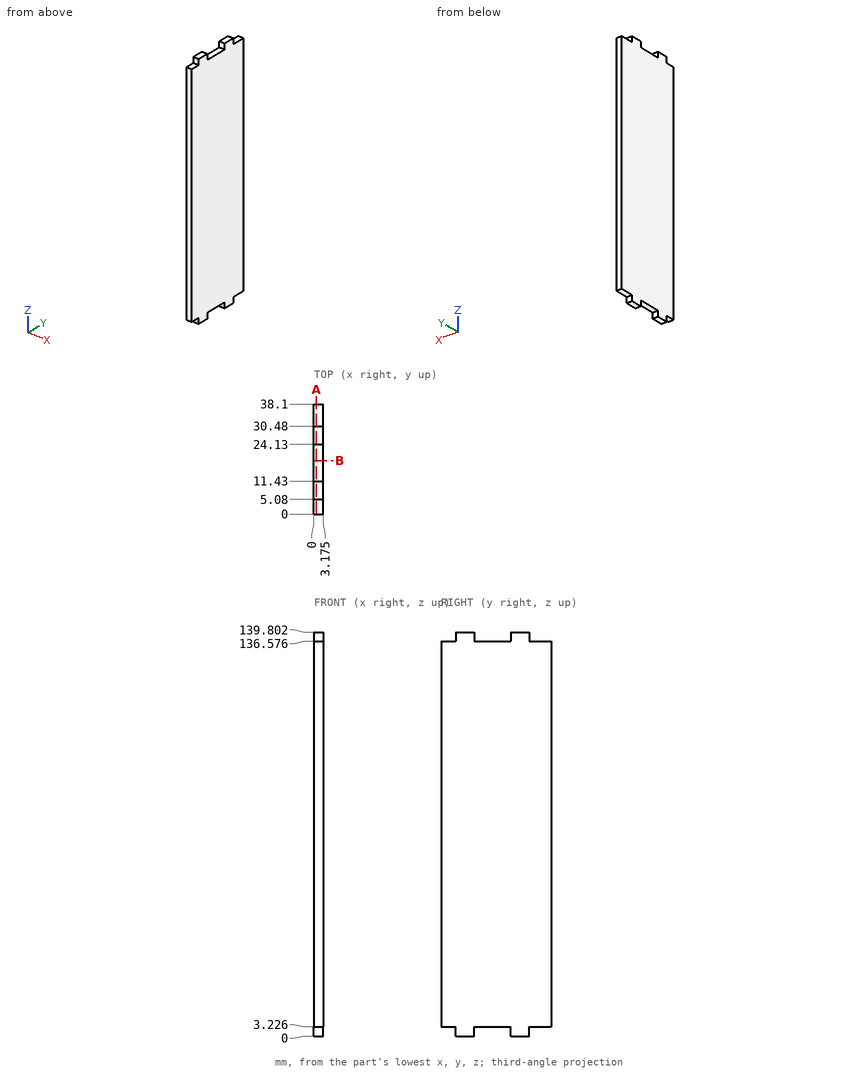
Geometry check sheet. Reference: drawing and pictorial views, mm from the part's lowest x, y, z. Give positions to 0.01 mm unless a question says otherwise; leave off trailing zeros. Loops run counter-clockwise (first coordinate to the right, second up) from the corner with the lowest first, then second, coordinate; pieces in that order, holes last. Notation, with made-up numbers: (61.5, -11.75) - (91.5, -11.75) arc R22 ccw to (91.5, 20.25) - close; hole circle Ø11 at (53, -19). An arc over 180 degrees is marked (long way). Use CSV: the item, a comma, the result in double quotes. Start each with the question number.
Q1. Go/stop test with flat-tipped pins: pin 1 Ø1.6 at (x, z) = (1.5, 2) entering from -Y; pin 2 Ø1 at (x, y) = (1.5, 14.5) entering from +Z; pin 3 Ø1.6 at (x, y) = (1.5, 17.5) entering from -Z. Record where each tip stops, or that it passes through.
Q2. Scan line: probe 1 along Z at (x, y) = (0.4, 21.5) (1 decimal). Record every from-to range of solid material in increasing order. Write a range as from..to.
Q3. Section check B-B, the plane y = 18.5. Record the cut outline in (x, z) (1 decimal).
Q4. Section check A-A, the plane x = 0.9. Record the cut outline in (y, z) (1 decimal), and give its area (3 significant figures).
Findings below:
1,pin 1,"stops at y = 5.08"
1,pin 2,"stops at z = 136.58"
1,pin 3,"stops at z = 3.23"
2,probe 1,"z = 3.2..136.6"
3,outline,"(0, 3.2) - (3.2, 3.2) - (3.2, 136.6) - (0, 136.6) - close"
4,outline,"(0, 3.2) - (5.1, 3.2) - (5.1, 0) - (11.4, 0) - (11.4, 3.2) - (24.1, 3.2) - (24.1, 0) - (30.5, 0) - (30.5, 3.2) - (38.1, 3.2) - (38.1, 136.6) - (30.5, 136.6) - (30.5, 139.8) - (24.1, 139.8) - (24.1, 136.6) - (11.4, 136.6) - (11.4, 139.8) - (5.1, 139.8) - (5.1, 136.6) - (0, 136.6) - close"
4,area,"5,160 mm^2"
